Design review of the part built by this model. Coordinates are the model's own, in mm. Face numbers are marked on the shaded views. A direction names the side the tool comes from. Coordinates: 2 decimals unless noted, no trailing zeros. Write each loop counter-clockwise with the first axis right and the second up, starting at its lowest first coordinate (ties: lowest second). Pieces come first, ordered by that corner, then holes. Notation, with made-up numbers: M 66.5,86.5 L 84.5,86.5 A34 cw 84.5,125.5 Z; hole C -23.75,65 d4. An arc over 180 degrees is marked long. Return JSON: item names as keys, results as strings. Group by question number.
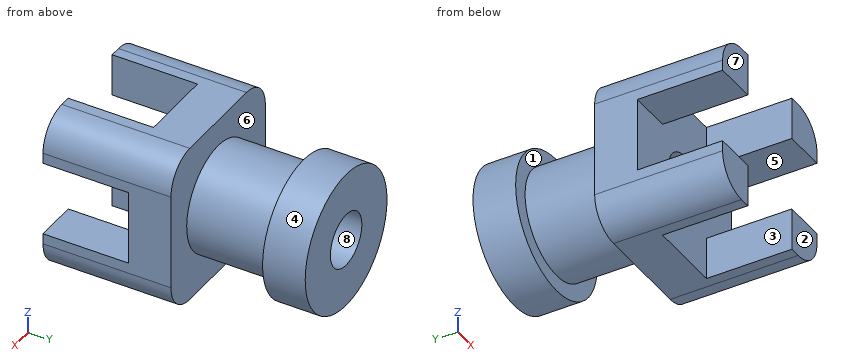
```python
from build123d import *

# Parameters (mm, degrees)
CROQUIS2_W              = 150
CROQUIS2_H              = 150
SALIENTE_EXTRUIR2_DEPTH = 40
CROQUIS3_W              = 40
CROQUIS3_H              = 40
SALIENTE_EXTRUIR3_DEPTH = 80
CROQUIS4_R              = 50
SALIENTE_EXTRUIR4_DEPTH = 120
CROQUIS5_R              = 25
CORTAR_EXTRUIR1_DEPTH   = 221
REDONDEO1_R             = 30
CROQUIS6_R              = 65
SALIENTE_EXTRUIR5_DEPTH = 40
CROQUIS7_R              = 25
CORTAR_EXTRUIR2_DEPTH   = 125


with BuildPart() as part:
    # Croquis2 → Saliente-Extruir2 (new body)
    with BuildSketch(Plane(origin=(0, 0, 0), x_dir=(1, 0, 0), z_dir=(0, 1, 0))):
        Rectangle(CROQUIS2_W, CROQUIS2_H)
    extrude(amount=SALIENTE_EXTRUIR2_DEPTH)

    # Croquis3 → Saliente-Extruir3 (add)
    with BuildSketch(Plane.XZ):
        with Locations((-55, 55)):
            Rectangle(CROQUIS3_W, CROQUIS3_H)
        with Locations((55, 55)):
            Rectangle(CROQUIS3_W, CROQUIS3_H)
        with Locations((-55, -55)):
            Rectangle(CROQUIS3_W, CROQUIS3_H)
        with Locations((55, -55)):
            Rectangle(CROQUIS3_W, CROQUIS3_H)
    extrude(amount=SALIENTE_EXTRUIR3_DEPTH)

    # Croquis4 → Saliente-Extruir4 (add)
    with BuildSketch(Plane(origin=(0, 40, 0), x_dir=(1, 0, 0), z_dir=(0, 1, 0))):
        with Locations(Location((0, 0, 0), (0, 0, 270))):
            Circle(CROQUIS4_R)
    extrude(amount=SALIENTE_EXTRUIR4_DEPTH)

    # Croquis5 → Cortar-Extruir1 (cut)
    with BuildSketch(Plane(origin=(0, 160, 0), x_dir=(1, 0, 0), z_dir=(0, 1, 0))):
        with Locations(Location((0, 0, 0), (0, 0, 270))):
            Circle(CROQUIS5_R)
    extrude(amount=-CORTAR_EXTRUIR1_DEPTH, mode=Mode.SUBTRACT)

    # Redondeo1
    redondeo1_edges = [part.edges().sort_by_distance(p)[0] for p in [
        (-75, -20, -75),
        (75, -20, -75),
        (75, -20, 75),
        (-75, -20, 75),
    ]]
    fillet(redondeo1_edges, radius=REDONDEO1_R)

    # Croquis6 → Saliente-Extruir5 (add)
    with BuildSketch(Plane(origin=(0, 160, 0), x_dir=(1, 0, 0), z_dir=(0, 1, 0))):
        with Locations(Location((0, 0, 0), (0, 0, 270))):
            Circle(CROQUIS6_R)
    extrude(amount=-SALIENTE_EXTRUIR5_DEPTH)

    # Croquis7 → Cortar-Extruir2 (cut)
    with BuildSketch(Plane(origin=(0, 160, 0), x_dir=(1, 0, 0), z_dir=(0, 1, 0))):
        with Locations(Location((0, 0, 0), (0, 0, 270))):
            Circle(CROQUIS7_R)
    extrude(amount=-CORTAR_EXTRUIR2_DEPTH, mode=Mode.SUBTRACT)


solid = part.part
```
Item 1: Machinability: for the marked faces 1, 2, 3, 4 and 5, which of the approach directions +Z, -Z, +X, -X, +Y, -Y give a long, thin tool a straight path to every point of the face, cutting with its end or side? Answer none if there is none.
Item 2: Add section A-A (y = -55). Write out the cut boundary in (x, z).
Item 3: The part is to be moulded in two halves that separate along Y. For the marked faces 6, 7 and 8, say which applies: pulls with the +Y half, pulls with the -Y half, needs draft (parallel to the pull), parting line crosses it, or undercut.
Item 4: For pin 1 (1.5 mm diameter, centred on y = 105.5, z = -2, fed in from +X); pin 2 (12 mm diameter, centred on x = 54.5, y = -36.5, fed in from -Z); pin 3 (8 mm diameter, centred on y = 63, z = -38, fed in from -X), all flat-tipped, find the tip position at first contact; note any pin that passes through.
Item 5: Add section C-C (z = 0). Write out the cut boundary in (x, y).
Item 6: Add section D-D (y = 84.5). Write out the cut boundary in (x, z), plus the area to 3 significant figures.
Item 7: Add section B-B (x = 0). Write out the cut boundary in (y, z), plus the area to 3 significant figures.
Item 8: For line 1 (Y direction, x = 8, z = -54.5); line 2 (Y direction, x = 42, z = -37); line 3 (X direction, y = 55, z = 0), list the stretches that pass through material, from the lowest coordinate up.
Geometry check:
{
 "1": {"face 1": "none", "face 2": "+Z, -Z, +X, -X, -Y", "face 3": "+Z, -Z, -Y", "face 4": "+Y", "face 5": "+X, -X, -Y"},
 "2": {"outline": "M -75,-45 A30 ccw -45,-75 L -35,-75 L -35,-35 L -75,-35 Z; M -75,35 L -35,35 L -35,75 L -45,75 A30 ccw -75,45 Z; M 35,-75 L 45,-75 A30 ccw 75,-45 L 75,-35 L 35,-35 Z; M 35,35 L 75,35 L 75,45 A30 ccw 45,75 L 35,75 Z"},
 "3": {"face 6": "undercut", "face 7": "pulls with the -Y half", "face 8": "needs draft"},
 "4": {"pin 1": "x = 49.98", "pin 2": "z = -74.8", "pin 3": "x = -36.66"},
 "5": {"outline": "M -75,0 L -25,0 L -25,160 L -65,160 L -65,120 L -50,120 L -50,40 L -75,40 Z; M 25,0 L 75,0 L 75,40 L 50,40 L 50,120 L 65,120 L 65,160 L 25,160 Z"},
 "6": {"outline": "C 0,0 d100; hole C 0,0 d50", "area": "5,890 mm^2"},
 "7": {"outline": "M 0,-75 L 40,-75 L 40,-50 L 120,-50 L 120,-65 L 160,-65 L 160,-25 L 0,-25 Z; M 0,25 L 160,25 L 160,65 L 120,65 L 120,50 L 40,50 L 40,75 L 0,75 Z", "area": "11,200 mm^2"},
 "8": {"line 1": "0 to 40, 120 to 160", "line 2": "-80 to 40, 120 to 160", "line 3": "-50 to -25, 25 to 50"}
}
